For this review, take the finished solid that the model builds, in its own axes (mm). A direction names the side the tool comes from. Round coordinates to 2 decimals unless told otherwise and drop trailing zeros. Write each loop counter-clockwise with the first axis right and the second up, starting at its lowest first coordinate (ties: lowest second). Pieces come first, ordered by that corner, then holes. Notation, with made-up numbers: M 44.5,19 L 92.5,19 A24 cw 92.5,54 Z; hole C 25.5,-17 d10. An arc over 180 degrees is marked long. Answer in a Markdown table with one row per item.
```python
from build123d import *

# Parameters (mm, degrees)
PAD_DEPTH             = 40
SKETCH004_R           = 150
POCKET001_DEPTH       = 28
THICKNESS_T           = -3
SKETCH003_R           = 27.5
SKETCH003_R_2         = 30
POCKET002_DEPTH       = 40.001
POCKET003_DEPTH       = 5
POLARPATTERN_COUNT    = 3
CHAMFER_ANGLE         = 60
CHAMFER_SIZE          = 1.1
CHAMFER003_SIZE       = 2
PAD004_DEPTH          = 2
POLARPATTERN002_COUNT = 3
CHAMFER004_SIZE       = 1.5


with BuildPart() as part:
    # Sketch002 → Pad (new body)
    with BuildSketch(Plane.XY.offset(22)):
        with BuildLine():
            ThreePointArc((-49.385877, 7.8125), (0, -50), (49.385877, 7.8125))
            Line((49.385877, 7.8125), (37.039408, 85.859375))
            ThreePointArc((37.039408, 85.859375), (0, 117.5), (-37.039408, 85.859375))
            Line((-49.385877, 7.8125), (-37.039408, 85.859375))
        make_face()
    extrude(amount=PAD_DEPTH)

    # Sketch004 (on Face5 of Pad) → Pocket001 (cut)
    with BuildSketch(Plane(origin=(0, 0, 22), x_dir=(1, 0, 0), z_dir=(0, 0, -1))):
        Circle(SKETCH004_R)
        with BuildLine():
            ThreePointArc((-32.10082, -85.078125), (0, -112.5), (32.10082, -85.078125))
            Line((32.10082, -85.078125), (44.447289, -7.03125))
            ThreePointArc((44.447289, -7.03125), (0, 45), (-44.447289, -7.03125))
            Line((-44.447289, -7.03125), (-32.10082, -85.078125))
        make_face(mode=Mode.SUBTRACT)
    extrude(amount=-POCKET001_DEPTH, mode=Mode.SUBTRACT)

    # Thickness
    thickness_openings = [part.faces().sort_by_distance(p)[0] for p in [
        (0, 29.917579, 22),
    ]]
    offset(amount=THICKNESS_T, openings=thickness_openings)

    # Sketch003 (on Face6 of Pad) → Pocket002 (cut, through all)
    with BuildSketch(Plane.XY.offset(62)):
        with Locations((0, 80)):
            Circle(SKETCH003_R)
        Circle(SKETCH003_R_2)
    extrude(amount=-POCKET002_DEPTH, mode=Mode.SUBTRACT)

    # Sketch005 (on Face4 of Pocket002) → Pocket003 (cut)
    with BuildSketch(Plane.XY.offset(62)):
        with BuildLine():
            ThreePointArc((0, -41.25), (2.25, -39), (0, -36.75))
            ThreePointArc((-12.56924, -34.533704), (-6.381571, -36.191685), (0, -36.75))
            ThreePointArc((-12.56924, -34.533704), (-21.733342, -33.592644), (-14.108331, -38.762321))
            ThreePointArc((-14.108331, -38.762321), (-7.162987, -40.62332), (0, -41.25))
        make_face()
    pocket003 = extrude(amount=-POCKET003_DEPTH, mode=Mode.SUBTRACT)

    # PolarPattern: Pocket003 ×3 about axis
    polarpattern_axis = Axis((0, 0, 62), (0, 0, 1))
    for i in range(1, POLARPATTERN_COUNT):
        add(pocket003.rotate(polarpattern_axis, i * 360 / POLARPATTERN_COUNT), mode=Mode.SUBTRACT)

    # Chamfer
    chamfer_edges = [part.edges().sort_by_distance(p)[0] for p in [
        (0, 114.5, 53),
    ]]
    chamfer_side = part.faces().sort_by_distance((0, 114.5, 56))[0]
    chamfer(chamfer_edges, length=CHAMFER_SIZE, angle=CHAMFER_ANGLE, reference=chamfer_side)

    # Chamfer003
    chamfer003_edges = [part.edges().sort_by_distance(p)[0] for p in [
        (0, -47, 59),
    ]]
    chamfer(chamfer003_edges, length=CHAMFER003_SIZE)

    # Sketch013 (on Face9 of Chamfer003) → Pad004 (join)
    with BuildSketch(Plane(origin=(0, 0, 59), x_dir=(1, 0, 0), z_dir=(0, 0, -1))):
        with BuildLine():
            ThreePointArc((-20.347983, 43.674473), (-25.727035, 32.139058), (-14.191621, 26.760006))
            Line((-15.645206, 30.753699), (-14.191621, 26.760006))
            ThreePointArc((-18.894398, 39.680779), (-21.733342, 33.592644), (-15.645206, 30.753699))
            Line((-20.347983, 43.674473), (-18.894398, 39.680779))
        make_face()
    pad004 = extrude(amount=PAD004_DEPTH)

    # PolarPattern002: Pad004 ×3 about axis
    polarpattern002_axis = Axis((0, 0, 59), (0, 0, -1))
    for i in range(1, POLARPATTERN002_COUNT):
        add(pad004.rotate(polarpattern002_axis, i * 360 / POLARPATTERN002_COUNT))

    # Chamfer004
    chamfer004_edges = [part.edges().sort_by_distance(p)[0] for p in [
        (-17.444958, 27.298151, 57),
        (-26.283288, 37.831262, 57),
        (-19.41828, -41.120134, 57),
        (-14.918413, -28.756853, 57),
        (45.320221, 3.743343, 57),
        (32.363372, 1.458701, 57),
    ]]
    chamfer(chamfer004_edges, length=CHAMFER004_SIZE)


solid = part.part
```
Q1. Machinability: for faces 5 (the face through (1.016, -41.988, 35.804)), 6 (the face through (-38.36, 45.51, 35.8)), 7 (the face through (39.209, 46.763, 53.542)), 8 (the face through (-1, 35, 62)), 9 (the face through (34.564, 12.485, 60.521)), which of the approach directions +Z, -Z, +X, -X, +Y, -Y give a long, thin tool a straight path to every point of the face, cutting with its end or side? Answer none if there is none.
Found:
| item | result |
|---|---|
| face 5 | -Z |
| face 6 | -Z, -X, +Y |
| face 7 | none |
| face 8 | +Z, +X, -X, +Y, -Y |
| face 9 | +Z, -Z |
Q2. Take a section at A-A (z = 39.5). State the section outline as (x, y) points.
Found:
| item | result |
|---|---|
| outline | M -44.45,7.03 A45 ccw long 44.45,7.03 L 32.1,85.08 A32.5 ccw -32.1,85.08 Z; hole M -41.48,6.56 A42 ccw long 41.48,6.56 L 29.14,84.61 A29.5 ccw -29.14,84.61 Z |
Q3. Insertion check: P1, Ø3, axis at x = -5.5, z = 41.5, coming from the -Y side; P2, Ø2, axis at x = -21, z = 57, coming from the -Y side; P3, Ø4, axis at x = -22, y = 38, coming from the -Z side. Each pin has a flat end and moves straight along its axis. Give the tip position at first contact, or say it passes through.
Found:
| item | result |
|---|---|
| P1 | y = -44.82 |
| P2 | y = -45.83 |
| P3 | z = 57 |
Q4. For probe 1 along X at (y, z) = (0, 56.15); probe 2 along X at (y, z) = (45.5, 38.5); probe 3 along Y at (x, z) = (20, 36.5), list the stretches that pass through material, from the lowest coordinate up.
Found:
| item | result |
|---|---|
| probe 1 | -50 to -47, 47 to 50 |
| probe 2 | -38.36 to -35.32, 35.32 to 38.36 |
| probe 3 | -40.31 to -36.93, 101.69 to 105.62 |
Q5. Mouldability with a two-part tool opening along X and no side actions: class faces 1 (the face through (-43.3, 46.29, 55.92)), 2 (the face through (1.088, -44.987, 35.804)), 3 (the face through (1.1, -45.39, 53.18)), 4 (the face through (2.25, -39.05, 60.52)) as +X half, -X half, draft (parallel to the pull), parting line (faces both ways), or undercut.
Found:
| item | result |
|---|---|
| face 1 | -X half |
| face 2 | parting line |
| face 3 | undercut |
| face 4 | undercut |
Q6. Take a section at B-B (x = -7). State how many separate pieces and enclosed holes the cut face has, then the cut area to 3 significant figures.
Found:
| item | result |
|---|---|
| separate pieces | 4 |
| enclosed holes | 0 |
| area | 410 mm² |
